```python
from build123d import *

# Parameters (mm, degrees)
SKETCH_1_R          = 16
SKETCH_1_R_2        = 7
EXTRUDE_1_DEPTH     = 3
SKETCH_2_R          = 9.5
SKETCH_2_R_2        = 7
EXTRUDE_2_DEPTH     = 10
SKETCH_3_R          = 2
CUT_EXTRUDE_1_DEPTH = 10


with BuildPart() as part:
    # 草图1 → 凸台-拉伸1 (new body)
    with BuildSketch(Plane.XY):
        Circle(SKETCH_1_R)
        Circle(SKETCH_1_R_2, mode=Mode.SUBTRACT)
    extrude(amount=EXTRUDE_1_DEPTH)

    # 草图2 → 凸台-拉伸2 (add)
    with BuildSketch(Plane.XY.offset(3)):
        Circle(SKETCH_2_R)
        Circle(SKETCH_2_R_2, mode=Mode.SUBTRACT)
    extrude(amount=EXTRUDE_2_DEPTH)

    # 草图3 → 切除-拉伸1 (cut)
    with BuildSketch(Plane.XY.offset(3)):
        with Locations((0, -12)):
            Circle(SKETCH_3_R)
        with Locations((-12, 0)):
            Circle(SKETCH_3_R)
        with Locations((0, 12)):
            Circle(SKETCH_3_R)
        with Locations((12, 0)):
            Circle(SKETCH_3_R)
    extrude(amount=-CUT_EXTRUDE_1_DEPTH, mode=Mode.SUBTRACT)


solid = part.part
```
For this review, take the finished solid that the model builds, in its own axes (mm). A direction names the side the tool comes from. Coordinates: 2 decimals unless noted, no trailing zeros. Write each loop counter-clockwise with the first axis right and the second up, starting at its lowest first coordinate (ties: lowest second). Pieces come first, ordered by that corner, then holes.
(1) Add section B-B on x = 12. Give the boundary of the cut face in (y, z), then the cut area to 3 significant figures.
(2) Add section D-D on y = -3.5. Give the boundary of the cut face in (x, z), then the cut area to 3 significant figures.
(3) For pin 1 Ø5 at (y, z) = (6.5, 9.5) entering from -X; pin 2 Ø4 at (y, z) = (10.5, 9.5) entering from +X, all flat-tipped, find the tip position at first contact; note any pin that passes through.
(4) Tool access review of faces 4 (the face through (0, -10, 2)), 5 (the face through (4.38, -8.43, 7.93)): name each direction out of +Z, -Z, +X, -X, +Y, -Y from which nothing blocks a thin tool from reaching the whole face with its end or side.
(5) The part is to be moulded in two halves that separate along X. For faces 1 (the face through (7, -7, 3)), 2 (the face through (-3.47, -15.62, 1.48)), 3 (the face through (10.4, -1.2, 1.5)), say which applies: +X half, -X half, draft (parallel to the pull), parting line (faces both ways), or undercut.
(6) Wall thickness on probe 1 along Y at (x, z) = (0, 1.75); probe 2 along X at (y, z) = (-5, 3.5); probe 3 along X at (y, z) = (-13.5, 1): over which ranges is each line inside the solid? List them lowest first.
(7) Add section A-A on y = 0. Give the boundary of the cut face in (x, z), then the cut area to 3 significant figures.
Answer sheet:
1. outline: (-10.58, 0) - (-2, 0) - (-2, 3) - (-10.58, 3) - close; (2, 0) - (10.58, 0) - (10.58, 3) - (2, 3) - close
1. area: 51.5 mm2
2. outline: (-15.61, 0) - (-6.06, 0) - (-6.06, 13) - (-8.83, 13) - (-8.83, 3) - (-15.61, 3) - close; (6.06, 0) - (15.61, 0) - (15.61, 3) - (8.83, 3) - (8.83, 13) - (6.06, 13) - close
2. area: 113 mm2
3. pin 1: stops at x = -8.62
3. pin 2: stops at x = 4.24
4. face 4: +Z, -Z
4. face 5: +Z
5. face 1: draft
5. face 2: parting line
5. face 3: undercut
6. probe 1: y = -16 to -14, -10 to -7, 7 to 10, 14 to 16
6. probe 2: x = -8.08 to -4.9, 4.9 to 8.08
6. probe 3: x = -8.59 to -1.32, 1.32 to 8.59
7. outline: (-16, 0) - (-14, 0) - (-14, 3) - (-16, 3) - close; (-10, 0) - (-7, 0) - (-7, 13) - (-9.5, 13) - (-9.5, 3) - (-10, 3) - close; (7, 0) - (10, 0) - (10, 3) - (9.5, 3) - (9.5, 13) - (7, 13) - close; (14, 0) - (16, 0) - (16, 3) - (14, 3) - close
7. area: 80.0 mm2
